Verification items for the finished model (mm, model axes). Face numbers are marked on the shaded views. Coordinates: 2 decimals unless noted, no trailing zeros. Write each loop counter-clockwise with the first axis right and the second up, starting at its lowest first coordinate (ties: lowest second). Pieces come first, ordered by that corner, then holes. Notation, with made-up numbers: M 31,79 L 88,79 A12 cw 88,90 Z; hole C 17,-5 d4. An arc over 180 degrees is marked long. Answer in a Markdown table with one row per item.
from build123d import *

# Parameters (mm, degrees)
SKETCH1_R               = 10
SKETCH1_R_2             = 7
MAIN_BODY_EXTRUDE_DEPTH = 2.5
F_2_OFFSET_BY           = 0.2
CHAMFER1_SIZE           = 1


with BuildPart() as part:
    # Sketch1 → Main Body Extrude (new, symmetric)
    with BuildSketch(Plane.XY):
        Circle(SKETCH1_R)
        Circle(SKETCH1_R_2, mode=Mode.SUBTRACT)
    extrude(amount=MAIN_BODY_EXTRUDE_DEPTH, both=True)

    # .2 Offset: a curved face moved outward by 0.2
    add(Solid.thicken(part.faces().sort_by_distance((-7, 0, 0))[0], F_2_OFFSET_BY))

    # Chamfer1
    chamfer1_edges = [part.edges().sort_by_distance(p)[0] for p in [
        (-10, 0, 2.5),
        (-10, 0, -2.5),
        (-6.8, 0, -2.5),
        (-6.8, 0, 2.5),
    ]]
    chamfer(chamfer1_edges, length=CHAMFER1_SIZE)


solid = part.part
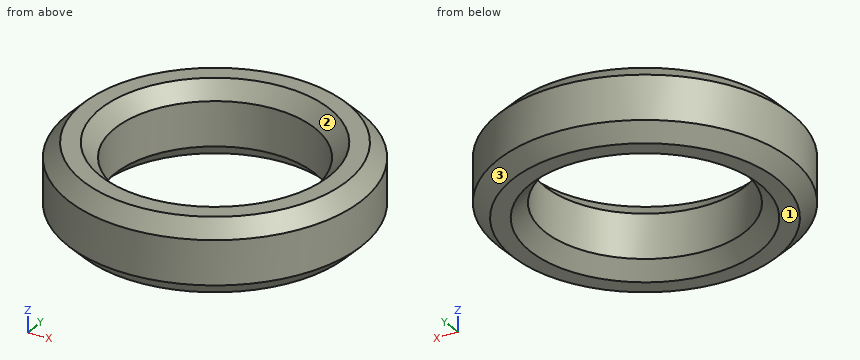
1) Sectioned sample at D-D (z = -0.7). Record the cut outline in (x, y), then the cut area to 3 significant figures.
Response values:
| item | result |
|---|---|
| outline | C 0,0 d20; hole C 0,0 d13.6 |
| area | 169 mm² |
2) Sectioned sample at C-C (z = -2). Record the cut outline in (x, y), then the cut area to 3 significant figures.
Response values:
| item | result |
|---|---|
| outline | C 0,0 d19; hole C 0,0 d14.6 |
| area | 116 mm² |
3) Depth check by flat-ended pin: pin 1 (2 mm diameter, centred on x = 1.5, y = 4, fed in from +Z); pin 2 (1 mm diameter, centred on x = -1.5, z = -1.5, fed in from -Y); pin 3 (1.5 mm diameter, centred on y = -1.5, z = -1, fed in from -X). Enter the tip coordinate at first touch or a pass-through.
Response values:
| item | result |
|---|---|
| pin 1 | passes through |
| pin 2 | stops at y = -9.95 |
| pin 3 | stops at x = -9.97 |
4) Sectioned sample at A-A (x = 0). Record the cut outline in (y, z).
Response values:
| item | result |
|---|---|
| outline | M -10,-1.5 L -9,-2.5 L -7.8,-2.5 L -6.8,-1.5 L -6.8,1.5 L -7.8,2.5 L -9,2.5 L -10,1.5 Z; M 6.8,-1.5 L 7.8,-2.5 L 9,-2.5 L 10,-1.5 L 10,1.5 L 9,2.5 L 7.8,2.5 L 6.8,1.5 Z |
5) Thickness scan on L1, parallel to Y at x = 0, z = -0.85; L2, parallel to Y at x = -1.5, z = 0.35; L3, parallel to X at y = 1.75, z = 0.8. Record the ranges inside material, lowest first. Write a range as [from, to].
Response values:
| item | result |
|---|---|
| L1 | y = [-10, -6.8], [6.8, 10] |
| L2 | y = [-9.89, -6.63], [6.63, 9.89] |
| L3 | x = [-9.85, -6.57], [6.57, 9.85] |
6) Release check for a two-part mould opening along Y. For the marked faces 1, 2 and 3 record: +Y half, -Y half, draft (parallel to the pull), parting line (faces both ways), or undercut.
Response values:
| item | result |
|---|---|
| face 1 | draft |
| face 2 | undercut |
| face 3 | parting line |
